For this review, take the finished solid that the model builds, in its own axes (mm). Face numbers are marked on the shaded views. A direction names the side the tool comes from. Coordinates: 2 decimals unless noted, no trailing zeros. Order: outer loops, then holes, each group sorted by start corner. A loop starts at its lowest first (then second) coordinate and runs counter-clockwise, first axis right, second up. Notation, with made-up numbers: (89.5, -13.75) -> (129.5, -13.75) arc R11 ccw to (129.5, -2.75) -> close; hole circle Ø3 at (12, 37). An arc over 180 degrees is marked (long way). Return JSON: item names as keys, results as strings. Group by question number.
Item 1: Take a section at C-C (y = -16.5). Write out the cut boundary in (x, z), then the cut area to 3 significant figures.
Item 2: Machinability: for the marked faces 4, 5 and 6, which of the approach directions +Z, -Z, +X, -X, +Y, -Y give a long, thin tool a straight path to every point of the face, cutting with its end or side? Answer none if there is none.
Item 3: Insertion check: pin 1 (7 mm diameter, centred on y = -12, z = 22, fed in from +X); pin 2 (7 mm diameter, centred on y = -12, z = 58, fed in from -X); pin 3 (1.5 mm diameter, centred on y = 18.5, z = 13, fed in from -X); pin 4 (3.5 mm diameter, centred on y = -12, z = 34, fed in from -X). Each pin has a flat end and moves straight along its axis. Give the tip position at first contact, or say it passes through.
Item 4: Draft analysis for pull direction Y (two halves, no side actions). For the marked faces 1, 2 and 3, state which applies: +Y half, -Y half, draft (parallel to the pull), parting line (faces both ways), or undercut.
Item 5: Take a section at A-A (y = 12). Count the separate pieces of the cut face and the enclosed holes in it, then the cut area to 3 significant figures.
Item 6: Take a section at B-B (x = -1.25). Write out the cut boundary in (y, z), then the cut area to 3 significant figures.
Item 7: For line 1 along Z through (x, y) = (-3.1, 24); line 2 along Z through (x, y) = (-9.45, -24); line 3 along X through (y, z) = (6, 27), list the stretches that pass through material, from the lowest coordinate up.
```python
from build123d import *

# Parameters (mm, degrees)
F0_W     = 4
F0_H     = 54
F1_DEPTH = 62
F2_DEPTH = 40
F4_R     = 2
F5_R     = 3
F6_DEPTH = 14.001
F8_DEPTH = 2
F9_DEPTH = 4
F10_R    = 1.99999


# Not quite as in the source:
# - a fillet or chamfer is up to 0.001 mm smaller than in the source, because OpenCascade refuses the exact size
# - a feature of the source that left no trace in its solid (it failed there, or was rolled back) is left out


with BuildPart() as f1:
    # F0 (on Top) → F1 (new body)
    with BuildSketch(Plane.XY):
        Polygon((4, -29), (4, 29), (-4, 29), (-4, 27), (-4, -27), (-4, -29), align=None)
        Rectangle(F0_W, F0_H, mode=Mode.SUBTRACT)
    extrude(amount=F1_DEPTH)

    # F0 (on Top) → F2 (join)
    with BuildSketch(Plane.XY):
        Polygon((-4, 27), (-4, 29), (-10, 29), (-10, 27), (-10, -27), (-10, -29), (-4, -29), (-4, -27), (-8, -27), (-8, 27), align=None)
    extrude(amount=F2_DEPTH)

    # F4
    f4_edges = [f1.edges().sort_by_distance(p)[0] for p in [
        (4, -29, 31),
        (4, 29, 31),
    ]]
    fillet(f4_edges, radius=F4_R)

    # F5 (on face) → F6 (cut, through all)
    with BuildSketch(Plane.YZ.offset(4)):
        with Locations((-24, 10)):
            Circle(F5_R)
        with Locations((-24, 22)):
            Circle(F5_R)
        with Locations((-24, 34)):
            Circle(F5_R)
        with Locations((-24, 46)):
            Circle(F5_R)
        with Locations((-12, 10)):
            Circle(F5_R)
        with Locations((-12, 22)):
            Circle(F5_R)
        with Locations((-12, 34)):
            Circle(F5_R)
        with Locations((-12, 46)):
            Circle(F5_R)
        with Locations((0, 10)):
            Circle(F5_R)
        with Locations((0, 22)):
            Circle(F5_R)
        with Locations((0, 34)):
            Circle(F5_R)
        with Locations((0, 46)):
            Circle(F5_R)
        with Locations((12, 10)):
            Circle(F5_R)
        with Locations((12, 22)):
            Circle(F5_R)
        with Locations((12, 34)):
            Circle(F5_R)
        with Locations((12, 46)):
            Circle(F5_R)
        with Locations((24, 10)):
            Circle(F5_R)
        with Locations((24, 22)):
            Circle(F5_R)
        with Locations((24, 34)):
            Circle(F5_R)
        with Locations((24, 46)):
            Circle(F5_R)
        with Locations((-24, 58)):
            Circle(F5_R)
        with Locations((-12, 58)):
            Circle(F5_R)
        with Locations((0, 58)):
            Circle(F5_R)
        with Locations((12, 58)):
            Circle(F5_R)
        with Locations((24, 58)):
            Circle(F5_R)
    extrude(amount=-F6_DEPTH, mode=Mode.SUBTRACT)

    # F7 (on face) → F8 (join)
    with BuildSketch(Plane.XY):
        with BuildLine():
            ThreePointArc((4, -31), (5.4142135624, -30.4142135624), (6, -29))
            Line((6, -29), (6, 29))
            ThreePointArc((6, 29), (5.4142135624, 30.4142135624), (4, 31))
            Line((4, 31), (-10, 31))
            ThreePointArc((-10, 31), (-11.4142135624, 30.4142135624), (-12, 29))
            Line((-12, 29), (-12, -29))
            ThreePointArc((-12, -29), (-11.4142135624, -30.4142135624), (-10, -31))
            Line((-10, -31), (4, -31))
        make_face()
    extrude(amount=-F8_DEPTH)

    # F9 (add): a face of the model
    f9_faces = [f1.faces().sort_by_distance(p)[0] for p in [
        (-10.957705074, -29.957705074, 0),
    ]]
    extrude(f9_faces, amount=F9_DEPTH)

    # F10 (radius 2 in the source; OpenCascade refuses exactly that, so slightly less here)
    f10_edges = [f1.edges().sort_by_distance(p)[0] for p in [
        (6, 0, -2),
        (-11.414214, -30.414214, -2),
        (-12, 0, -2),
        (-11.414214, 30.414214, -2),
        (-3, 31, -2),
        (5.414214, 30.414214, -2),
        (5.414214, -30.414214, -2),
        (-4, -29, 51),
        (-4, 29, 51),
        (-10, -29, 22),
        (-10, 29, 22),
        (-3, -31, -2),
    ]]
    fillet(f10_edges, radius=F10_R)


solid = f1.part
```
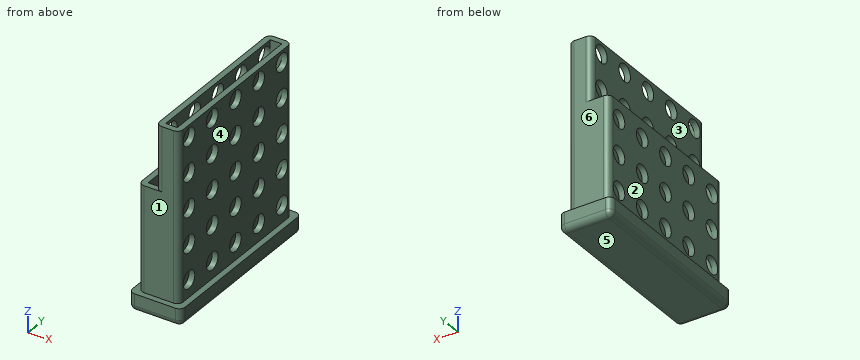
Findings below:
{
 "1": {"outline": "(-12, 0) arc R2 ccw to (-10, -2) -> (4, -2) arc R2 ccw to (6, 0) -> (6, 4) -> (4, 4) -> (4, 62) -> (2, 62) -> (2, 0) -> (-2, 0) -> (-2, 62) -> (-4, 62) -> (-4, 0) -> (-8, 0) -> (-8, 40) -> (-10, 40) -> (-10, 4) -> (-12, 4) -> close", "area": "378 mm2"},
 "2": {"face 4": "+Z, +X, +Y, -Y", "face 5": "-Z, +X, -X, +Y, -Y", "face 6": "+Z, +X, -X, +Y"},
 "3": {"pin 1": "stops at x = 4", "pin 2": "stops at x = -4", "pin 3": "stops at x = -10", "pin 4": "passes through"},
 "4": {"face 1": "-Y half", "face 2": "draft", "face 3": "undercut"},
 "5": {"separate pieces": "14", "enclosed holes": "0", "area": "222 mm2"},
 "6": {"outline": "(-31, 0) arc R2 ccw to (-29, -2) -> (29, -2) arc R2 ccw to (31, 0) -> (31, 4) -> (29, 4) -> (29, 62) -> (27, 62) -> (27, 0) -> (-27, 0) -> (-27, 62) -> (-29, 62) -> (-29, 4) -> (-31, 4) -> close", "area": "386 mm2"},
 "7": {"line 1": "z = -2 to 7, 13 to 19, 25 to 31, 37 to 43, 49 to 55, 61 to 62", "line 2": "z = -2 to 7, 13 to 19, 25 to 31, 37 to 40", "line 3": "x = -10 to -8, -4 to -2, 2 to 4"}
}
